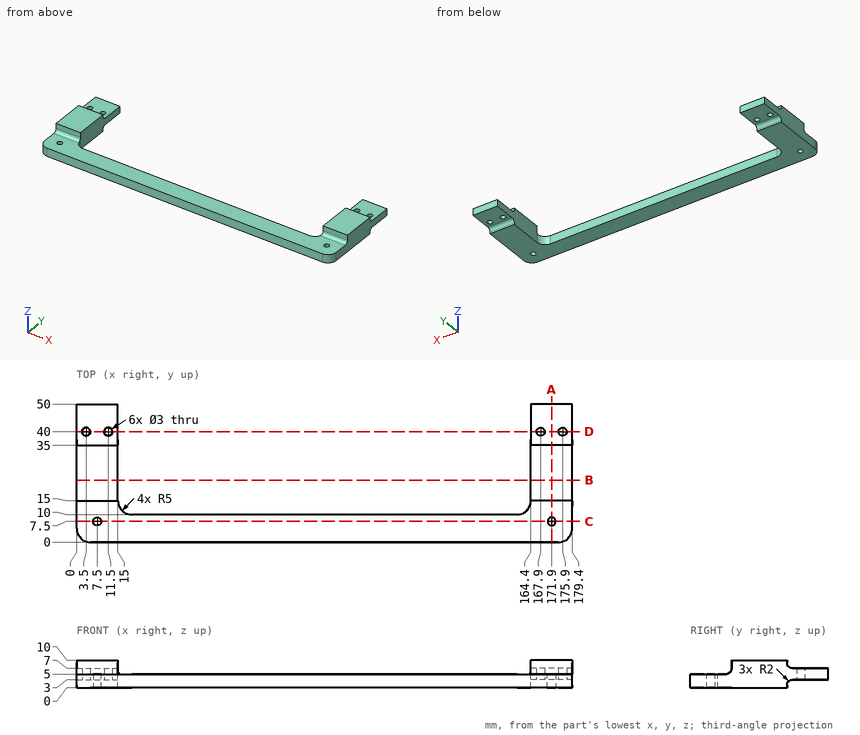
Source: three-view drawing plus pictorial views. Frame: mm from the lowest corner of the part. Coordinates: 2 decimals unless noted, no trailing zeros. Loops run counter-clockwise (first coordinate to the right, second up) from the corner with the lowest first, then second, coordinate; pieces in that order, holes last. Notation, with made-up numbers: M 0.25,4.25 L 12.25,4.25 A21 cw 12.25,21.25 Z; hole C 38.5,-32.5 d10. An arc over 180 degrees is marked long. Use CSV: the item, a comma, the result in double quotes.
(1) Cut plane B-B on y = 22.5. Return loops of the section in (x, z).
Answers follow:
outline,"M 0,0 L 15,0 L 15,10 L 0,10 Z; M 164.4,0 L 179.4,0 L 179.4,10 L 164.4,10 Z"
(2) Contact query for flat-ended pins moving along their axis: pin 1 (2.5 mm diameter, centred on x = 174, z = 9, fed in from -Y); pin 2 (0.8 mm diameter, centred on x = 6, z = 0.5, fed in from +Y); pin 3 (6.5 mm diameter, centred on x = 63, y = 6.5, fed in from +Z). Output: stop coordinate, or through.
Answers follow:
pin 1,"y = 15"
pin 2,"y = 35"
pin 3,"z = 5"
(3) Cut plane C-C on y = 7.5. Return loops of the section in (x, z).
Answers follow:
outline,"M 0,0 L 6,0 L 6,5 L 0,5 Z; M 9,0 L 170.4,0 L 170.4,5 L 9,5 Z; M 173.4,0 L 179.4,0 L 179.4,5 L 173.4,5 Z"
(4) Cut plane D-D on y = 40. Return loops of the section in (x, z), and give its area (3 significant figures).
Answers follow:
outline,"M 0,3 L 2,3 L 2,7 L 0,7 Z; M 5,3 L 10,3 L 10,7 L 5,7 Z; M 13,3 L 15,3 L 15,7 L 13,7 Z; M 164.4,3 L 166.4,3 L 166.4,7 L 164.4,7 Z; M 169.4,3 L 174.4,3 L 174.4,7 L 169.4,7 Z; M 177.4,3 L 179.4,3 L 179.4,7 L 177.4,7 Z"
area,"72.0 mm²"
(5) Line query: line 1 (X direction, y = 40, z = 3.5); line 2 (X direction, y = 18.5, z = 4.5); line 3 (Z direction, x = 10, y = 13). Output: solid intervals per line, ascending. Write a range as [from, to].
Answers follow:
line 1,"[0, 2], [5, 10], [13, 15], [164.4, 166.4], [169.4, 174.4], [177.4, 179.4]"
line 2,"[0, 15], [164.4, 179.4]"
line 3,"[0, 5]"
(6) Cut plane A-A on x = 171.9. Return loops of the section in (y, z), and give its area (3 significant figures).
Answers follow:
outline,"M 0,0 L 6,0 L 6,5 L 0,5 Z; M 9,0 L 35,0 L 35,1 A2 cw 37,3 L 50,3 L 50,7 L 37,7 A2 cw 35,9 L 35,10 L 15,10 L 15,7 A2 cw 13,5 L 9,5 Z"
area,"323 mm²"
